For this review, take the finished solid that the model builds, in its own axes (mm). A direction names the side the tool comes from. Round coordinates to 2 decimals unless told otherwise and drop trailing zeros. Loops run counter-clockwise (first coordinate to the right, second up) from the corner with the lowest first, then second, coordinate; pieces in that order, holes last. Notation, with made-up numbers: (-13.5, 18) -> (17.5, 18) arc R15 cw to (17.5, 43) -> close; hole circle Ø9 at (-35.5, -38). An arc over 180 degrees is marked (long way). Use one line per item in the form item = value. Start each with the question number.
Autodesk Fusion 360 part; units mm, degrees
sketch "スケッチ1" plane through (0, 0, 0) normal (1, 0, 0) x (0, 0, -1)
  circle A0 centre (0, 0) radius 27
  dimension "d1" = 54
extrude "押し出し1" add sketch "スケッチ1" along normal blind 1.2
sketch "スケッチ2" plane through (1.2, 0, 0) normal (1, 0, 0) x (0, 0, -1)
  circle A0 centre (0, 0) radius 27
  circle A1 centre (0, 0) radius 19
  dimension "d4" = 38
extrude "押し出し2" add sketch "スケッチ2" along normal blind 3.8 contours A1
sketch "スケッチ7" plane through (5, 0, 0) normal (1, 0, 0) x (0, 0, -1)
  circle A0 centre (0, 0) radius 19
  arc A1 (0, 20) -> (-13.9054, 14.375) centre (0, 0) ccw
  arc A2 (-17.3011, -10.0336) -> (-5.4591, -19.2405) centre (0, 0) ccw
  arc A3 (19.3599, -5.0193) -> (17.3316, 9.9807) centre (0, 0) ccw
  line L0 (17.3316, 9.9807) -> (0, 0)
  line L1 (0, 0) -> (19.3599, -5.0193)
  line L2 (0, 20) -> (0, 0)
  line L3 (-13.9054, 14.375) -> (0, 0)
  line L4 (-17.3011, -10.0336) -> (0, 0)
  line L5 (-5.4591, -19.2405) -> (0, 0)
  dimension "d10" = 20
  dimension "d11" = 20
  dimension "d12" = 20
  dimension "d13" = 15
  dimension "d14" = 15
  dimension "d15" = 15
extrude "押し出し3" add sketch "スケッチ7" against normal blind 1 contours A0 A3 L0 L1 | A0 A1 L2 L3 | A0 A2 L4 L5
sketch "スケッチ12" plane through (1.2, 0, 0) normal (1, 0, 0) x (0, 0, -1)
  circle A0 centre (0, 0) radius 19
  circle A1 centre (0, 0) radius 27
  arc A2 (-24.592, -5.0724) -> (-22.0631, -9.3178) centre (-23, -7) ccw
  arc A3 (-21.3514, -8.9648) -> (-23.2882, -4.3834) centre (-22.5544, -6.7733) ccw
  line L0 (-22.0631, -9.3178) -> (-21.3514, -8.9648)
  line L1 (-24.592, -5.0724) -> (-23.2882, -4.3834)
  dimension "d38" = 2.5
  dimension "d39" = 2.5
  dimension "d62" = 0.5
  dimension "d63" = 1.476
extrude "押し出し10" cut sketch "スケッチ12" against normal blind 11 contours A2 A3 L0 L1
sketch "スケッチ8" plane through (0, 0, 0) normal (-1, 0, 0) x (0, 0, 1)
  circle A0 centre (0, 0) radius 27
  circle A1 centre (0, 0) radius 20
  arc A2 (23.2882, -4.3834) -> (21.3514, -8.9648) centre (22.5544, -6.7733) ccw
  line L0 (23.2882, -4.3834) -> (24.592, -5.0724)
  arc A3 (22.0631, -9.3178) -> (24.592, -5.0724) centre (23, -7) ccw
  line L1 (22.0631, -9.3178) -> (21.3514, -8.9648)
  dimension "d18" = 40
extrude "押し出し4" add sketch "スケッチ8" along normal blind 10 contours A1
sketch "スケッチ9" plane through (5, 0, 0) normal (1, 0, 0) x (0, 0, -1)
  arc A0 (16.465, 9.4817) -> (0, 19) centre (0, 0) ccw
  line L0 (0, 19) -> (0, 20)
  arc A1 (0, 20) -> (-13.9054, 14.375) centre (0, 0) ccw
  line L1 (-13.9054, 14.375) -> (-13.2101, 13.6563)
  arc A2 (-13.2101, 13.6563) -> (-16.436, -9.5319) centre (0, 0) ccw
  line L2 (-16.436, -9.5319) -> (-17.3011, -10.0336)
  arc A3 (-17.3011, -10.0336) -> (-5.4591, -19.2405) centre (0, 0) ccw
  line L3 (-5.4591, -19.2405) -> (-5.1861, -18.2785)
  arc A4 (-5.1861, -18.2785) -> (18.3919, -4.7683) centre (0, 0) ccw
  line L4 (18.3919, -4.7683) -> (19.3599, -5.0193)
  arc A5 (19.3599, -5.0193) -> (17.3316, 9.9807) centre (0, 0) ccw
  line L5 (17.3316, 9.9807) -> (16.465, 9.4817)
  circle A6 centre (0, 0) radius 15
  dimension "d21" = 30
extrude "押し出し5" cut sketch "スケッチ9" against normal blind 14 contours A6
sketch "スケッチ11" plane through (-9, 0, 0) normal (1, 0, 0) x (0, 0, -1)
  circle A0 centre (0, 0) radius 15
  line L0 (-2.5, 2.5) -> (2.5, 2.5)
  line L1 (2.5, 2.5) -> (2.5, -2.5)
  line L2 (2.5, -2.5) -> (-2.5, -2.5)
  line L3 (-2.5, -2.5) -> (-2.5, 2.5)
  line L4 (5, 10) -> (10, 10)
  line L5 (10, 10) -> (10, 5)
  line L6 (10, 5) -> (5, 5)
  line L7 (5, 5) -> (5, 10)
  line L8 (-10, 10) -> (-5, 10)
  line L9 (-5, 10) -> (-5, 5)
  line L10 (-5, 5) -> (-10, 5)
  line L11 (-10, 5) -> (-10, 10)
  line L12 (-10, -5) -> (-5, -5)
  line L13 (-5, -5) -> (-5, -10)
  line L14 (-5, -10) -> (-10, -10)
  line L15 (-10, -10) -> (-10, -5)
  line L16 (5, -5) -> (10, -5)
  line L17 (10, -5) -> (10, -10)
  line L18 (10, -10) -> (5, -10)
  line L19 (5, -10) -> (5, -5)
  dimension "d42" = 5
  dimension "d43" = 2.5
  dimension "d44" = 2.5
  dimension "d45" = 5
  dimension "d46" = 5
  dimension "d47" = 5
  dimension "d48" = 5
  dimension "d49" = 5
  dimension "d50" = 5
  dimension "d51" = 5
  dimension "d52" = 5
  dimension "d53" = 5
  dimension "d54" = 5
  dimension "d55" = 5
  dimension "d56" = 5
  dimension "d57" = 5
  dimension "d58" = 5
  dimension "d59" = 5
extrude "押し出し11" cut sketch "スケッチ11" against normal blind 5 contours L0 L1 L2 L3 | L4 L5 L6 L7 | L8 L9 L10 L11 | L12 L13 L14 L15 | L16 L17 L18 L19
Item 1: Take a section at A-A on y = 0. Give the boundary of the cut face in (x, z).
Item 2: Draft analysis for pull direction Y (two halves, no side actions). For faces 4 (the cylindrical face through (4.51, 18.58, 7.4)), 5 (the cylindrical face through (-1.902, 0.66, 14.985)), 6 (the flat face through (-10, 0, 4)), state which applies: +Y half, -Y half, draft (parallel to the pull), parting line (faces both ways), or undercut.
Item 3: Take a section at D-D on x = -1.5. Give the boundary of the cut face in (y, z), plus the area to 3 significant figures.
Item 4: Take a section at C-C on z = -8.5. Give the boundary of the cut face in (x, y).
Item 5: Wall thickness on line 1 (Y direction, x = -4.5, z = 0); line 2 (Z direction, x = 4.25, y = -4.5); line 3 (X direction, y = -20.5, z = 7): over which ranges is each line inside the solid? List them lowest first.
Item 6: Take a section at B-B on y = 6. Give the boundary of the cut face in (x, z), plus the area to 3 significant figures.
Item 7: Machinability: for faces 1 (the cylindrical face through (3.07, -18.84, 2.47)), 2 (the flat face through (0, -20, -4)), 3 (the flat face through (0.608, -4.733, 23.949)), which of the approach directions +Z, -Z, +X, -X, +Y, -Y give a long, thin tool a straight path to every point of the face, cutting with its end or side? Answer none if there is none.
Item 8: For P1, Ø1.5, axis at x = 0, y = -3, coming from the +Z side; P2, Ø2, axis at y = 20.5, z = -7.5, coming from the +X side; P3, Ø1.1, axis at x = -9.5, y = 6.5, coming from the -Z side, all flat-tipped, find the tip position at first contact; note any pin that passes through.
Results:
q1.outline = (-10, -20) -> (0, -20) -> (0, -27) -> (1.2, -27) -> (1.2, -19) -> (4, -19) -> (4, -20) -> (5, -20) -> (5, -15) -> (-9, -15) -> (-9, -2.5) -> (-10, -2.5) -> close; (-10, 2.5) -> (-9, 2.5) -> (-9, 15) -> (5, 15) -> (5, 19) -> (1.2, 19) -> (1.2, 27) -> (0, 27) -> (0, 20) -> (-10, 20) -> close
q2.face_4 = +Y half
q2.face_5 = undercut
q2.face_6 = draft
q3.outline = circle Ø40 at (0, 0); hole circle Ø30 at (0, 0)
q3.area = 550 mm2
q4.outline = (-10, -18.1) -> (0, -18.1) -> (0, -25.63) -> (1.2, -25.63) -> (1.2, -16.99) -> (5, -16.99) -> (5, -12.36) -> (-9, -12.36) -> (-9, -10) -> (-10, -10) -> close; (-10, -5) -> (-9, -5) -> (-9, 5) -> (-10, 5) -> close; (-10, 10) -> (-9, 10) -> (-9, 12.36) -> (5, 12.36) -> (5, 16.99) -> (1.2, 16.99) -> (1.2, 25.63) -> (0, 25.63) -> (0, 18.1) -> (-10, 18.1) -> close
q5.line_1 = -20 to -15, 15 to 20
q5.line_2 = -19.49 to -14.31, 14.31 to 18.46
q5.line_3 = 0 to 1.2
q6.outline = (-10, -19.08) -> (0, -19.08) -> (0, -26.32) -> (1.2, -26.32) -> (1.2, -18.03) -> (4, -18.03) -> (4, -19.08) -> (5, -19.08) -> (5, -13.75) -> (-9, -13.75) -> (-9, -10) -> (-10, -10) -> close; (-10, -5) -> (-9, -5) -> (-9, 5) -> (-10, 5) -> close; (-10, 10) -> (-9, 10) -> (-9, 13.75) -> (5, 13.75) -> (5, 18.03) -> (1.2, 18.03) -> (1.2, 26.32) -> (0, 26.32) -> (0, 19.08) -> (-10, 19.08) -> close
q6.area = 188 mm2
q7.face_1 = none
q7.face_2 = -X
q7.face_3 = +X, -X
q8.P1 = 26.91
q8.P2 = 1.2
q8.P3 = -19.09
